Input: part model. Units: mm. Frame: model coordinates. A direction names the side the tool comes from. Round coordinates to 2 decimals unless told otherwise and drop trailing zeros. Loops run counter-clockwise (first coordinate to the right, second up) from the corner with the lowest first, then second, coordinate; pieces in that order, holes last. Notation, with made-up numbers: M 11.25,74 L 69.25,74 A37 cw 69.25,112 Z; hole C 37,4.5 d11. An arc over 180 degrees is marked long. Return JSON: item names as keys, results as strings. Group by question number.
1) Section D-D (z = 169). Count the separate pieces of the cut face and the enclosed holes in it, plus the area to 3 significant figures.
2) Section B-B (y = 0). Output: boundary loops of the cut face in (x, z).
3) Material intervals for line 1 (X direction, y = -5, z = 417.5); line 2 (X direction, y = -227.5, z = 180); line 3 (Z direction, x = 28, y = 104.5), sorted ascending. Write a range as from..to.
4) Section A-A (z = -30). Output: boundary loops of the cut face in (x, y), plus the area to 3 significant figures.
5) Mould query, pull axis Y, two halves, no side actions, for faces 5 (the face through (176, -193.408, 97)), 6 (the face through (195, -186, 300)), 7 (the face through (-179, -198.408, 97)). Classes: +Y half, -Y half, draft (parallel to the pull), parting line (faces both ways), or undercut.
6) Contact query for flat-ended pins moving along their axis: P1, Ø17.5, axis at y = 170, z = 183.5, coming from the +X side; P2, Ø8, axis at y = -199, z = 313.5, coming from the -X side; P3, Ø6, axis at x = 101, y = 46, coming from the +Z side; P4, Ø12, axis at x = -179, y = 184, coming from the +Z side. Output: stop coordinate, or through.
7) Access query for faces 1 (the face through (-178, 198.408, 103)), 2 (the face through (-195, -187, 300)), 3 (the face through (178, -198.408, 97)), 4 (the face through (-3, 3, 0)). Directions: +Z, -Z, +X, -X, +Y, -Y. A direction counts if a zero-diameter tool reaches every point of the face in a straight line with its end or side. Return the directions, or none.
from build123d import *

# Parameters (mm, degrees)
F0_R          = 253
F1_DEPTH      = 500
F2_R          = 50
F3_T          = -3
F5_DEPTH      = 300
F5_DEPTH_BACK = 100


with BuildPart() as f1:
    # F0 (on Top) → F1 (new body)
    with BuildSketch(Plane.XY):
        Circle(F0_R)
    extrude(amount=F1_DEPTH)

    # F2
    f2_edges = [f1.edges().sort_by_distance(p)[0] for p in [
        (-253, 0, 0),
    ]]
    fillet(f2_edges, radius=F2_R)

    # F3
    f3_openings = [f1.faces().sort_by_distance(p)[0] for p in [
        (0, 0, 500),
    ]]
    offset(amount=F3_T, openings=f3_openings)

    # F4 (on Top) → F5 (join, two sides)
    with BuildSketch(Plane.XY) as f5_sk:
        Polygon((-158.408357, 193.408357), (-158.408357, 198.408357), (-198.408357, 198.408357), (-198.408357, 158.408357), (-193.408357, 158.408357), (-193.408357, 193.408357), align=None)
        Polygon((158.408357, 198.408357), (158.408357, 193.408357), (193.408357, 193.408357), (193.408357, 158.408357), (198.408357, 158.408357), (198.408357, 198.408357), align=None)
        Polygon((198.408357, -198.408357), (198.408357, -158.408357), (193.408357, -158.408357), (193.408357, -193.408357), (158.408357, -193.408357), (158.408357, -198.408357), align=None)
        Polygon((-193.408357, -158.408357), (-198.408357, -158.408357), (-198.408357, -198.408357), (-158.408357, -198.408357), (-158.408357, -193.408357), (-193.408357, -193.408357), align=None)
    extrude(amount=F5_DEPTH)
    extrude(f5_sk.sketch, amount=-F5_DEPTH_BACK)


solid = f1.part
Returned:
{
 "1": {"separate pieces": "1", "enclosed holes": "5", "area": "6,170 mm^2"},
 "2": {"outline": "M -253,50 A50 ccw -203,0 L 203,0 A50 ccw 253,50 L 253,500 L 250,500 L 250,50 A47 cw 203,3 L -203,3 A47 cw -250,50 L -250,500 L -253,500 Z"},
 "3": {"line 1": "x = -252.95..-249.95, 249.95..252.95", "line 2": "x = -110.69..-103.65, 103.65..110.69", "line 3": "z = 0..3"},
 "4": {"outline": "M -198.41,-198.41 L -158.41,-198.41 L -158.41,-193.41 L -193.41,-193.41 L -193.41,-158.41 L -198.41,-158.41 Z; M -198.41,158.41 L -193.41,158.41 L -193.41,193.41 L -158.41,193.41 L -158.41,198.41 L -198.41,198.41 Z; M 158.41,-198.41 L 198.41,-198.41 L 198.41,-158.41 L 193.41,-158.41 L 193.41,-193.41 L 158.41,-193.41 Z; M 158.41,193.41 L 193.41,193.41 L 193.41,158.41 L 198.41,158.41 L 198.41,198.41 L 158.41,198.41 Z", "area": "1,500 mm^2"},
 "5": {"face 5": "undercut", "face 6": "draft", "face 7": "-Y half"},
 "6": {"P1": "stops at x = 198.41", "P2": "stops at x = -161.2", "P3": "stops at z = 3", "P4": "stops at z = 500"},
 "7": {"face 1": "+Z, -Z, -X, +Y", "face 2": "+Z, -X, -Y", "face 3": "+Z, -Z, +X, -Y", "face 4": "-Z"}
}
